Verification items for the finished model (mm, model axes). Round coordinates to 2 decimals unless told otherwise and drop trailing zeros. Write each loop counter-clockwise with the first axis right and the second up, starting at its lowest first coordinate (ties: lowest second). Pieces come first, ordered by that corner, then holes. Notation, with made-up numbers: (69.25, 52) -> (112.25, 52) arc R21 cw to (112.25, 72) -> close; hole circle Ø6 at (58.5, 32). An arc over 180 degrees is marked (long way). Answer as a JSON object with one key per item and string values. Group by question number.
(1) Sectioned sample at C-C on x = -1. Record the cut outline in (y, z).
(2) Sectioned sample at D-D on z = 0.55. Record the cut outline in (x, y).
(3) Gauge pin test, flat end, axial feed: pin 1 Ø2 at (x, y) = (-0.5, 5) entering from +Z. Record the tip position at first contact, or that the pin passes through.
(4) Sectioned sample at B-B on y = 9.75. Record the cut outline in (x, z).
(5) Draft check along X on faces 1 (the face through (0, 6, 1)), 2 (the face through (1, 13, 1)), 3 (the face through (-2.165, 6, 3)). Enter one of: released by +X, released by -X, zero draft, split by the parting line, or undercut.
(6) Scan lines: L1, parallel to X at y = 9.5, z = 2.5; L2, parallel to Z at x = 0.45, y = 4; L3, parallel to Z at x = 1.05, y = 9.75. Record each from-to range of solid material in increasing order. Write a range as from..to.
(7) Sectioned sample at A-A on z = 2.5. Record the cut outline in (x, y).
Autodesk Inventor part; units mm, degrees
ref_plane "YZ Plane" through (0, 0, 0) normal (1, 0, 0) x (0, 1, 0)
ref_plane "XZ Plane" through (0, 0, 0) normal (0, 1, 0) x (-1, 0, 0)
ref_plane "XY Plane" through (0, 0, 0) normal (0, 0, 1) x (1, 0, 0)
sketch "Эскиз1" plane through (0, 0, 0) normal (0, 1, 0) x (-1, 0, 0)
  line L0 (0, 0) -> (0, 5)
  line L1 (0, 0) -> (-2.1651, 1.25)
  line L2 (-2.1651, 1.25) -> (-2.1651, 3.75)
  line L3 (-2.1651, 3.75) -> (0, 5)
  line L4 (0, 5) -> (2.1651, 3.75)
  line L5 (2.1651, 3.75) -> (2.1651, 1.25)
  line L6 (2.1651, 1.25) -> (0, 0)
  circle A0 centre (0, 2.5) radius 1.5
  dimension "d0" = 5
  dimension "d1" = 3
extrude "Выдавливание1" add sketch "Эскиз1" along normal blind 13 contours L1 L2 L3 L0 A0 | L0 A0 L4 L5 L6
thread "Резьба1"
properties part number "rack_25"
Computed values:
{
 "1": {"outline": "(0, 0.58) -> (13, 0.58) -> (13, 1.38) -> (0, 1.38) -> close; (0, 3.62) -> (13, 3.62) -> (13, 4.42) -> (0, 4.42) -> close"},
 "2": {"outline": "(-0.95, 0) -> (0.95, 0) -> (0.95, 13) -> (-0.95, 13) -> close"},
 "3": {"pin 1": "z = 5"},
 "4": {"outline": "(-2.17, 1.25) -> (0, 0) -> (2.17, 1.25) -> (2.17, 3.75) -> (0, 5) -> (-2.17, 3.75) -> close; hole circle Ø3 at (0, 2.5)"},
 "5": {"face 1": "undercut", "face 2": "zero draft", "face 3": "released by -X"},
 "6": {"L1": "-2.17..-1.5, 1.5..2.17", "L2": "0.26..1.07, 3.93..4.74", "L3": "0.61..1.43, 3.57..4.39"},
 "7": {"outline": "(-2.17, 0) -> (-1.5, 0) -> (-1.5, 13) -> (-2.17, 13) -> close; (1.5, 0) -> (2.17, 0) -> (2.17, 13) -> (1.5, 13) -> close"}
}
